Could you check a few things on this drawing? It's one solid part, dimensions in mm from its lowest x, y, z. A direction names the side the tool comes from. Give positions to 0.01 mm unless a question says otherwise; leave off trailing zeros. Order: outer loops, then holes, each group sorted by start corner. A loop starts at its lowest first (then second) coordinate and runs counter-clockwise, first axis right, second up. Notation, with made-up numbers: (-29.5, -23.75) -> (4.5, -23.75) arc R21 cw to (4.5, 14.25) -> close; hole circle Ø7 at (-35, -23.5). An arc over 180 degrees is marked (long way). Answer as a JSON object with one key per item and string values.
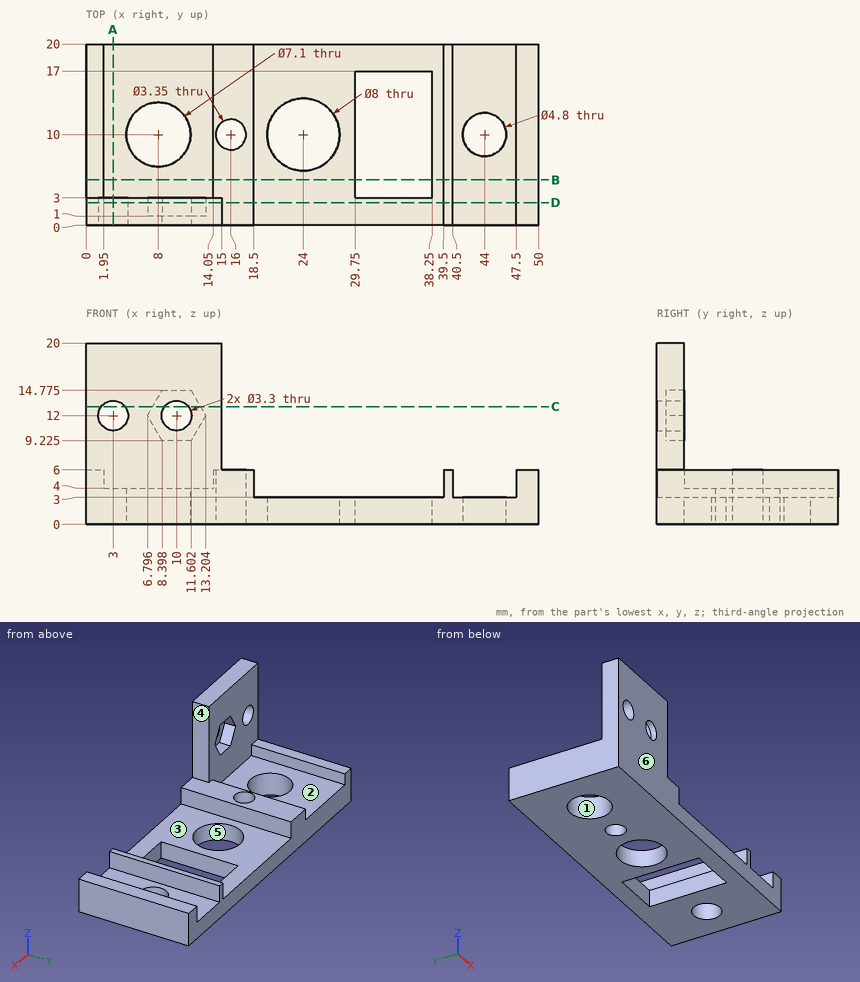
1. If we section it at A-A on x = 3: Please give me the cut outline in (y, z), then the cut area to 3 significant figures.
Worked answers:
{"outline": "(0, 0) -> (20, 0) -> (20, 4) -> (3, 4) -> (3, 10.35) -> (0, 10.35) -> close; (0, 13.65) -> (3, 13.65) -> (3, 20) -> (0, 20) -> close", "area": "118 mm²"}
2. If we section it at D-D on y = 2.5: Count the separate pieces of the cut face and the enclosed holes in it, then the cut area to 3 significant figures.
Worked answers:
{"separate pieces": "1", "enclosed holes": "2", "area": "391 mm²"}
3. Please list where these lines run through material, in increasing order: L1, parallel to Y at x = 8, z = 2.15; L2, parallel to Y at x = 44, z = 1.1; L3, parallel to Z at x = 15, y = 6.
Worked answers:
{"L1": "0 to 6.45, 13.55 to 20", "L2": "0 to 7.6, 12.4 to 20", "L3": "0 to 6"}
4. If we section it at C-C on z = 13: Please give me the cut outline in (x, y), then the cut area to 3 significant figures.
Worked answers:
{"outline": "(0, 0) -> (1.69, 0) -> (1.69, 3) -> (0, 3) -> close; (4.31, 0) -> (8.69, 0) -> (8.69, 1) -> (7.37, 1) -> (7.37, 3) -> (4.31, 3) -> close; (11.31, 0) -> (15, 0) -> (15, 3) -> (12.63, 3) -> (12.63, 1) -> (11.31, 1) -> close", "area": "24.0 mm²"}
5. If we section it at B-B on y = 5: Please give me the cut outline in (x, z).
Worked answers:
{"outline": "(0, 0) -> (29.75, 0) -> (29.75, 3) -> (18.5, 3) -> (18.5, 6) -> (14.05, 6) -> (14.05, 4) -> (1.95, 4) -> (1.95, 6) -> (0, 6) -> close; (38.25, 0) -> (50, 0) -> (50, 6) -> (47.5, 6) -> (47.5, 3) -> (40.5, 3) -> (40.5, 6) -> (39.5, 6) -> (39.5, 3) -> (38.25, 3) -> close"}
6. If we mould it in two halves opening along Y, with no side actions, what happens to the marked faces 4, 5 and 6? For each: +Y half, -Y half, draft (parallel to the pull), parting line (faces both ways), or undercut.
Worked answers:
{"face 4": "draft", "face 5": "undercut", "face 6": "-Y half"}
7. For the marked faces 1, 2 and 3, which set-ups out of +Z, -Z, +X, -X, +Y, -Y let a thin tool reach every point of the face, with its end or its side?
Worked answers:
{"face 1": "+Z, -Z", "face 2": "+Z, +Y", "face 3": "+Z, +Y, -Y"}
8. Will these pins go through, and if not, where does the flat tip stop? pin 1 Ø8 at (x, z) = (6, 12) entering from +Y; pin 2 Ø12 at (x, z) = (41.5, 12.5) entering from +Y; pin 3 Ø0.6 at (x, y) = (0.5, 12.5) entering from +Z; pin 4 Ø2.5 at (y, z) = (1.5, 13.5) entering from +X.
Worked answers:
{"pin 1": "y = 3", "pin 2": "through", "pin 3": "z = 6", "pin 4": "x = 15"}
